Autodesk Inventor part; units mm, degrees
ref_plane "YZ Plane" through (0, 0, 0) normal (1, 0, 0) x (0, 1, 0)
ref_plane "XZ Plane" through (0, 0, 0) normal (0, 1, 0) x (-1, 0, 0)
ref_plane "XY Plane" through (0, 0, 0) normal (0, 0, 1) x (1, 0, 0)
sketch "Sketch1" plane through (0, 0, 0) normal (0, 0, 1) x (1, 0, 0)
  line L0 (0, 0) -> (-7, 0)
  line L1 (-7, 0) -> (-11.5963, 3.8567)
  line L2 (-11.5963, 3.8567) -> (-24, 148.3252)
  line L3 (-24, 148.3252) -> (-24, 216.3252)
  line L4 (-24, 216.3252) -> (-11.5963, 251.1842)
  line L5 (-11.5963, 251.1842) -> (-7, 255.0409)
  line L6 (-7, 255.0409) -> (0, 255.0409)
  line L7 (0, 255.0409) -> (0, 0)
  line L8 (0, 6) -> (-4, 6)
  line L9 (-4, 6) -> (-4, 21)
  line L10 (-4, 21) -> (0, 21)
  line L11 (-5.5, 46) -> (-2.5, 46)
  line L12 (-2.5, 46) -> (-2.5, 125.6208)
  line L13 (-2.5, 125.6208) -> (-14.0543, 145.6334)
  line L14 (-14.0543, 145.6334) -> (-5.5, 46)
  line L15 (0, 249.0409) -> (-5, 249.0409)
  line L16 (-5, 249.0409) -> (-7.135, 243.0409)
  line L17 (-7.135, 243.0409) -> (0, 238.9899)
  line L18 (-8.7779, 238.224) -> (-2.5, 234.6596)
  line L19 (-2.5, 234.6596) -> (-2.5, 220.224)
  line L20 (-2.5, 220.224) -> (-15.1828, 220.224)
  line L21 (-15.1828, 220.224) -> (-8.7779, 238.224)
  line L22 (0, 131.2907) -> (-14, 155.5394)
  arc A0 (0, 204) -> (0, 196) centre (0, 200) ccw
  circle A1 centre (-7, 200) radius 1.5
  line L23 (0, 0) -> (7, 0)
  line L24 (7, 0) -> (11.5963, 3.8567)
  line L25 (11.5963, 3.8567) -> (24, 148.3252)
  line L26 (24, 148.3252) -> (24, 216.3252)
  line L27 (24, 216.3252) -> (11.5963, 251.1842)
  line L28 (11.5963, 251.1842) -> (7, 255.0409)
  line L29 (7, 255.0409) -> (0, 255.0409)
  line L30 (0, 6) -> (4, 6)
  line L31 (4, 6) -> (4, 21)
  line L32 (4, 21) -> (0, 21)
  line L33 (5.5, 46) -> (2.5, 46)
  line L34 (2.5, 46) -> (2.5, 125.6208)
  line L35 (2.5, 125.6208) -> (14.0543, 145.6334)
  line L36 (14.0543, 145.6334) -> (5.5, 46)
  line L37 (0, 249.0409) -> (5, 249.0409)
  line L38 (5, 249.0409) -> (7.135, 243.0409)
  line L39 (7.135, 243.0409) -> (0, 238.9899)
  line L40 (8.7779, 238.224) -> (2.5, 234.6596)
  line L41 (2.5, 234.6596) -> (2.5, 220.224)
  line L42 (2.5, 220.224) -> (15.1828, 220.224)
  line L43 (15.1828, 220.224) -> (8.7779, 238.224)
  line L44 (0, 131.2907) -> (14, 155.5394)
  arc A2 (0, 196) -> (0, 204) centre (0, 200) ccw
  circle A3 centre (-16.5993, 116.8252) radius 2
  circle A4 centre (16.5993, 116.8252) radius 2
  circle A5 centre (-8.5, 27) radius 2
  circle A6 centre (8.5, 27) radius 2
  line L45 (0, 200) -> (-10, 200)
  line L46 (0, 204) -> (-14, 204)
  line L47 (0, 196) -> (-14, 196)
  circle A7 centre (-4.9497, 195.0503) radius 1.5
  circle A8 centre (0, 193) radius 1.5
  circle A9 centre (4.9497, 195.0503) radius 1.5
  circle A10 centre (7, 200) radius 1.5
  circle A11 centre (0, 207) radius 1.5
  line L48 (-14, 155.5394) -> (-14, 176.2907)
  arc A12 (-14, 176.2907) -> (0, 161.3241) centre (1, 176.2907) ccw
  line L49 (14, 155.5394) -> (14, 176.2907)
  arc A13 (0, 161.3241) -> (14, 176.2907) centre (-1, 176.2907) ccw
  point P0 (0, 155.5394)
  dimension "d0" = 7
  dimension "d1" = 6
  dimension "d2" = 145
  dimension "d3" = 68
  dimension "d4" = 37
  dimension "d5" = 48
  dimension "d8" = 140
  dimension "d9" = 140
  dimension "d10" = 15
  dimension "d11" = 6
  dimension "d12" = 4
  dimension "d13" = 3
  dimension "d14" = 5
  dimension "d15" = 25
  dimension "d17" = 100
  dimension "d19" = 5
  dimension "d20" = 28
  dimension "d21" = 150
  dimension "d29" = 6
  dimension "d32" = 6
  dimension "d33" = 4
  dimension "d38" = 3
  dimension "d42" = 4
  dimension "d43" = 31.5
  dimension "d45" = 5
  dimension "d46" = 4
  dimension "d47" = 17
  dimension "d48" = 6
  dimension "d51" = 200
  dimension "d54" = 3
  dimension "d56" = 14
  dimension "d57" = 8
  dimension "d58" = 7
  dimension "d61" = 180
  dimension "d63" = 5
  dimension "d64" = 5
  dimension "d65" = 100
  dimension "d66" = 7
  dimension "d67" = 5
  dimension "d68" = 18
  dimension "d69" = 15
  dimension "d70" = 15
  dimension "d71" = 45
extrude "Extrusion1" add sketch "Sketch1" along normal mid plane 4 contours L0 L1 L2 L3 L4 L5 L6 L7 L15 L16 L17 A11 A0 A8 A12 L48 L22 L10 L9 L8 | L7 L30 L31 L32 L44 L49 A13 A8 A2 A11 L39 L38 L37 L29 L28 L27 L26 L25 L24 L23 | A8 L7 | L7 A8 | A11 L7 | L7 A11
extrude "Extrusion2" cut sketch "Sketch1" along normal mid plane 10 contours A8 L7 | L7 A8 | A11 L7 | L7 A11
properties part number "Leg_part3"
Can you work these out from the model? Positions are in its coordinate system, mm. A direction names the side the tool comes from. Give positions to 0.01 mm unless a question says otherwise; leave off trailing zeros. Order: outer loops, then holes, each group sorted by start corner. A loop starts at its lowest first (then second) coordinate and runs counter-clockwise, first axis right, second up. Notation, with made-up numbers: M 59.25,15.25 L 74.25,15.25 A15 ccw 74.25,20.25 Z; hole C 54.5,43.25 d6. An arc over 180 degrees is marked long. One line per item, written item: value.
1) On a 3-axis mill with a long thin cutter (end or side, diameter ignored), from which of +Z, -Z, +X, -X, +Y, -Y can I reach the whole of each face in a straight line? I mean faces 1 (the face through (-2.5, 228, 0)), 2 (the face through (0, 255.041, 0)). Say none if no direction works.
Answer sheet:
face 1: +Z, -Z
face 2: +Z, -Z, +X, -X, +Y
2) For P1, Ø4, axis at x = -4.95, y = 195.05, coming from the +Z side, with a flat end and sliding along its axis, tell me the tip position at first contact or that it passes through.
Answer sheet:
P1: stops at z = 2
3) Please list where these lines run through material, in increasing order: line 1 along X through (y, z) = (200, -1); line 2 along X through (y, z) = (88.5, 0.6); line 3 along X through (y, z) = (81.5, -0.9).
Answer sheet:
line 1: x = -24 to -8.5, -5.5 to -4, 4 to 5.5, 8.5 to 24
line 2: x = -18.86 to -9.15, -2.5 to 2.5, 9.15 to 18.86
line 3: x = -18.26 to -8.55, -2.5 to 2.5, 8.55 to 18.26
4) I want a section at C-C, the plane z = -1.1. Count the separate pieces of the cut face and the enclosed holes in it, plus the area to 3 significant figures.
Answer sheet:
separate pieces: 1
enclosed holes: 18
area: 7,290 mm^2
5) I want a section at A-A, the plane y = 226. List the corners of the cut face in (x, z) for me, plus the area to 3 significant figures.
Answer sheet:
outline: M -20.56,-2 L -13.13,-2 L -13.13,2 L -20.56,2 Z; M -2.5,-2 L 2.5,-2 L 2.5,2 L -2.5,2 Z; M 13.13,-2 L 20.56,-2 L 20.56,2 L 13.13,2 Z
area: 79.4 mm^2
6) We'd pull the mould along Y, two halves only. Please class faces 3 (the face through (9, 220.224, 0)), 4 (the face through (0, 129, 2)), 5 (the face through (-17.885, 233.511, -0.028)), 6 (the face through (-5.683, 236.467, 0.028)): released by +Y, released by -Y, zero draft, split by the parting line, or undercut.
Answer sheet:
face 3: undercut
face 4: zero draft
face 5: released by +Y
face 6: undercut
7) I want a section at D-D, the plane y = 106. List the corners of the cut face in (x, z) for me, plus the area to 3 significant figures.
Answer sheet:
outline: M -20.37,-2 L -10.65,-2 L -10.65,2 L -20.37,2 Z; M -2.5,-2 L 2.5,-2 L 2.5,2 L -2.5,2 Z; M 10.65,-2 L 20.37,-2 L 20.37,2 L 10.65,2 Z
area: 97.7 mm^2
8) I want a section at B-B, the plane y = 141. List the corners of the cut face in (x, z) for me.
Answer sheet:
outline: M -23.37,-2 L -13.66,-2 L -13.66,2 L -23.37,2 Z; M -11.38,-2 L -5.61,-2 L -5.61,2 L -11.38,2 Z; M 5.61,-2 L 11.38,-2 L 11.38,2 L 5.61,2 Z; M 13.66,-2 L 23.37,-2 L 23.37,2 L 13.66,2 Z
